Build history of the part. All positions in model axes, mm. Face numbers are marked on the shaded views. A direction names the side the tool comes from. Round coordinates to 2 decimals unless told otherwise and drop trailing zeros. Write each loop counter-clockwise with the first axis right and the second up, starting at its lowest first coordinate (ties: lowest second). Pieces come first, ordered by that corner, then holes. Notation, with made-up numbers: M 45,65.25 L 61,65.25 A23 ccw 61,78.25 Z; hole C 60,-35.75 d2. An arc over 180 degrees is marked long. Write item = value, one per line. Start each with the question number.
Q1. Band-saw the part on C-C on x = 13.5. Write the cut outline in (y, z), plus the area to 3 significant figures.
Q2. Band-saw the part on D-D on x = 2. Write the cut outline in (y, z).
Q3. Probe L1, parallel to Y at x = 9.75, z = 0; L2, parallel to Z at x = 7, y = -1; L3, parallel to X at y = 3.25, z = 0.5. List the from-to ranges inside material, lowest first.
Q4. Pull direction Y, two halves, no side cores. Call the marked faces 3, 4 and 5: released by +Y, released by -Y, zero draft, split by the parting line, or undercut.
Q5. Drop flat-ended pins along their axis: P1, Ø1, axis at x = 7, z = 3, coming from the +Y side; P2, Ø3, axis at x = 13, z = 3, coming from the +Y side. Give the stop position or say it passes through.
Q6. Band-saw the part on A-A on y = 0. Write the cut outline in (x, z), plus the area to 3 significant figures.
Q7. Tool access for the marked faces 1 and 2: list every direction of +Z, -Z, +X, -X, +Y, -Y with a clear straight run to the whole face (end or side of a thin tool).
```python
from build123d import *

# Parameters (mm, degrees)
F2_R           = 0.5
F4_D           = 4
F4_CSINK_D     = 6
F4_CSINK_ANGLE = 90


with BuildPart() as f1:
    # F0 (on Front) → F1 (revolve)
    with BuildSketch(Plane.XZ):
        Polygon((0, 3.75), (0, 0), (16, 0), (16, 3), (2.5, 3), (2.5, 3.75), align=None)
    revolve(axis=Axis((8, 0, 0), (-1, 0, 0)))

    # F2
    f2_edges = [f1.edges().sort_by_distance(p)[0] for p in [
        (0, 0, -3.75),
    ]]
    fillet(f2_edges, radius=F2_R)

    # F4 (through all)
    with Locations(Plane(origin=(0, 0, 0), x_dir=(0, -1, 0), z_dir=(-1, 0, 0))):
        with Locations((0, 0)):
            CounterSinkHole(F4_D / 2, F4_CSINK_D / 2, counter_sink_angle=F4_CSINK_ANGLE)


solid = f1.part
```
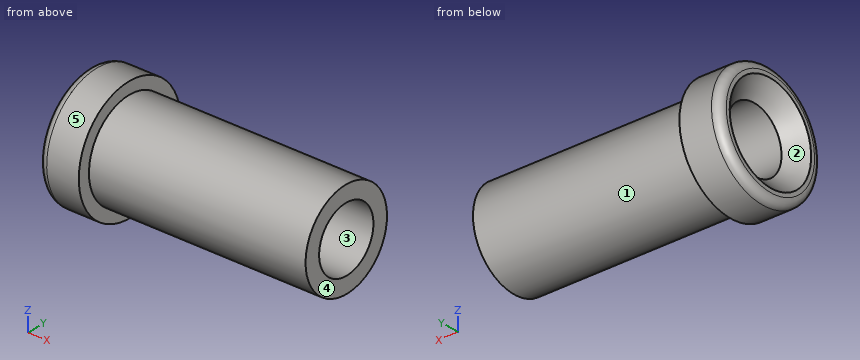
Conclusion:
q1.outline = C 0,0 d6; hole C 0,0 d4
q1.area = 15.7 mm^2
q2.outline = C 0,0 d7.5; hole C 0,0 d4
q3.L1 = -3 to -2, 2 to 3
q3.L2 = -2.83 to -1.73, 1.73 to 2.83
q3.L3 = 0 to 2.5
q4.face_3 = undercut
q4.face_4 = zero draft
q4.face_5 = split by the parting line
q5.P1 = 1.66
q5.P2 = 2.6
q6.outline = M 0,-3.25 A0.5 ccw 0.5,-3.75 L 2.5,-3.75 L 2.5,-3 L 16,-3 L 16,-2 L 1,-2 L 0,-3 Z; M 0,3 L 1,2 L 16,2 L 16,3 L 2.5,3 L 2.5,3.75 L 0.5,3.75 A0.5 ccw 0,3.25 Z
q6.area = 34.6 mm^2
q7.face_1 = +X
q7.face_2 = -X
